Geometry: final body of the model. Coordinates: model frame, mm. Face numbers are marked on the shaded views. A direction names the side the tool comes from. Give positions to 0.01 mm unless a question says otherwise; leave off trailing zeros. Write each loop counter-clockwise with the first axis right and the second up, starting at its lowest first coordinate (ties: lowest second). Pieces come first, ordered by that corner, then holes.
Q1. Pin query (flat end, axial travel): pin 1 (1.3 mm diameter, centred on x = 6.35, y = -10, fed in from -Z). Return the tip coordinate at first contact, or that it passes through.
Q2. Cut plane D-D on x = -6.35. Return the cut outline in (y, z), plus the area to 3 significant figures.
Q3. Cut plane B-B on z = 1.95. Return the cut outline in (x, y), plus the area to 3 significant figures.
Q4. Reachability of the marked faces 4 and 5 from +Z, -Z, +X, -X, +Y, -Y: full face, straight path, thin tool, end or side. Return the list, or none.
Q5. Cut plane C-C on y = -10. Return the cut outline in (x, z), plus the area to 3 significant figures.
Q6. Line query: L1, parallel to Y at x = 6.35, z = 1.55; L2, parallel to Y at x = 0.5, z = 1.65; L3, parallel to Y at x = -6, z = 2. Output: solid intervals per line, ascending.
Q7. Cut plane A-A on x = 0.5. Return the cut outline in (y, z), plus the area to 3 significant figures.
Q8. Draft query along Y for the marked faces 1, 2 and 3. Return one class per face: pulls with the +Y half, pulls with the -Y half, needs draft (parallel to the pull), parting line crosses it, or undercut.
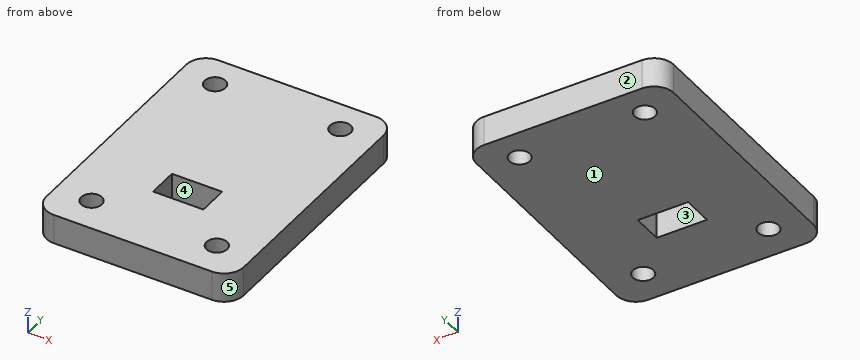
```python
from build123d import *

# Parameters (mm, degrees)
CROQUIS1_W              = 20
CROQUIS1_H              = 27
SALIENTE_EXTRUIR1_DEPTH = 3
CROQUIS2_W              = 5.1
CROQUIS2_H              = 3.1
CORTAR_EXTRUIR1_DEPTH   = 10
CROQUIS3_R              = 1.05
CORTAR_EXTRUIR2_DEPTH   = 10
REDONDEO1_R             = 2


with BuildPart() as part:
    # Croquis1 → Saliente-Extruir1 (new body)
    with BuildSketch(Plane.XY):
        Rectangle(CROQUIS1_W, CROQUIS1_H)
    extrude(amount=SALIENTE_EXTRUIR1_DEPTH)

    # Croquis2 → Cortar-Extruir1 (cut)
    with BuildSketch(Plane.XY.offset(3)):
        with Locations((0, -4.5)):
            Rectangle(CROQUIS2_W, CROQUIS2_H)
    extrude(amount=-CORTAR_EXTRUIR1_DEPTH, mode=Mode.SUBTRACT)

    # Croquis3 → Cortar-Extruir2 (cut)
    with BuildSketch(Plane.XY.offset(3)):
        with Locations((-6.35, 10.32)):
            Circle(CROQUIS3_R)
        with Locations((6.35, 10.32)):
            Circle(CROQUIS3_R)
        with Locations((6.35, -10)):
            Circle(CROQUIS3_R)
        with Locations((-6.35, -10)):
            Circle(CROQUIS3_R)
    extrude(amount=-CORTAR_EXTRUIR2_DEPTH, mode=Mode.SUBTRACT)

    # Redondeo1
    redondeo1_edges = [part.edges().sort_by_distance(p)[0] for p in [
        (10, -13.5, 1.5),
        (-10, -13.5, 1.5),
        (-10, 13.5, 1.5),
        (10, 13.5, 1.5),
    ]]
    fillet(redondeo1_edges, radius=REDONDEO1_R)


solid = part.part
```
Data:
1. pin 1: passes through
2. outline: (-13.5, 0) - (-11.05, 0) - (-11.05, 3) - (-13.5, 3) - close; (-8.95, 0) - (9.27, 0) - (9.27, 3) - (-8.95, 3) - close; (11.37, 0) - (13.5, 0) - (13.5, 3) - (11.37, 3) - close
2. area: 68.4 mm2
3. outline: (-10, -11.5) arc R2 ccw to (-8, -13.5) - (8, -13.5) arc R2 ccw to (10, -11.5) - (10, 11.5) arc R2 ccw to (8, 13.5) - (-8, 13.5) arc R2 ccw to (-10, 11.5) - close; hole circle Ø2.1 at (-6.35, -10); hole circle Ø2.1 at (-6.35, 10.32); hole (-2.55, -6.05) - (2.55, -6.05) - (2.55, -2.95) - (-2.55, -2.95) - close; hole circle Ø2.1 at (6.35, -10); hole circle Ø2.1 at (6.35, 10.32)
3. area: 507 mm2
4. face 4: +Z, -Z
4. face 5: +Z, -Z, +X, -Y
5. outline: (-10, 0) - (-7.4, 0) - (-7.4, 3) - (-10, 3) - close; (-5.3, 0) - (5.3, 0) - (5.3, 3) - (-5.3, 3) - close; (7.4, 0) - (10, 0) - (10, 3) - (7.4, 3) - close
5. area: 47.4 mm2
6. L1: y = -13.5 to -11.05, -8.95 to 9.27, 11.37 to 13.5
6. L2: y = -13.5 to -6.05, -2.95 to 13.5
6. L3: y = -13.5 to -10.99, -9.01 to 9.33, 11.31 to 13.5
7. outline: (-13.5, 0) - (-6.05, 0) - (-6.05, 3) - (-13.5, 3) - close; (-2.95, 0) - (13.5, 0) - (13.5, 3) - (-2.95, 3) - close
7. area: 71.7 mm2
8. face 1: needs draft
8. face 2: pulls with the +Y half
8. face 3: undercut
